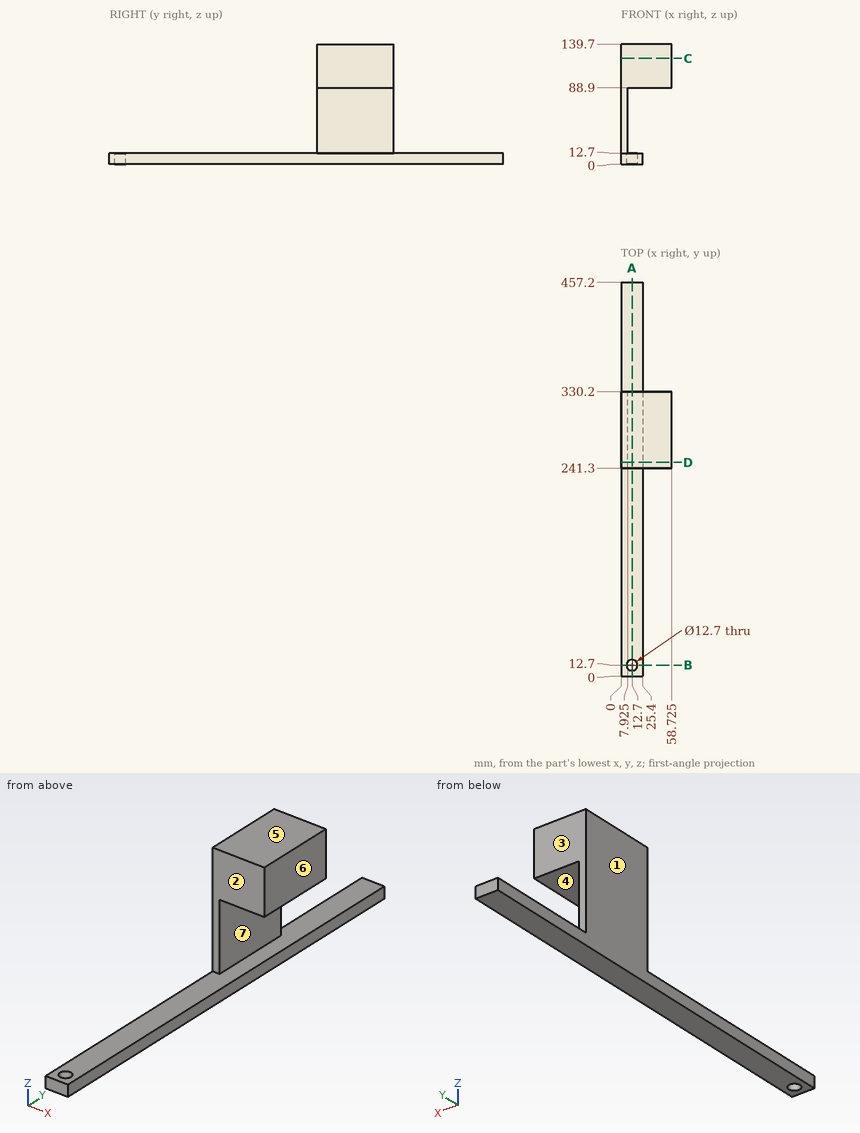
Answer from the drawing. Dimensions are ordinates in mm from the lowest x, y and z of the part. A direction names the side the tool comes from. Coordinates: 2 decimals unless noted, no trailing zeros. Write each loop counter-clockwise with the first axis right and the second up, starting at its lowest first coordinate (ties: lowest second). Pieces come first, ordered by that corner, then holes. Notation, with made-up numbers: M 46.25,7.5 L 84.25,7.5 A15 cw 84.25,27.5 Z; hole C 84.5,7.5 d5. An arc over 180 degrees is marked long. Use one line per item in the form item = value. Start each with the question number.
1. Each of these flat-tipped pins is pushed along its axis until it touches: P1, Ø4, axis at x = 27.5, z = 113.5, coming from the -Y side; P2, Ø1, axis at x = 52, z = 120.5, coming from the +Y side; P3, Ø6.5, axis at y = 216.5, z = 8.5, coming from the +X side; P4, Ø11.5, axis at x = 12.7, y = 12.7, coming from the -Z side. Where does it stop, or does it pass through?
2. The mould has two halves that part along Z. Classify the marked faces 4, 5, 6 and 7: released by +Z, released by -Z, zero draft, split by the parting line, or undercut.
3. A tool of negligible diameter and unlimited length cuts with its end or side. For the marked faces 1, 2 and 3, from which of +Z, -Z, +X, -X, +Y, -Y can it reach the whole face along a straight path? Write none if from no direction.
4. The part is cut by section A-A (x = 12.7). Give the vertices of the cut face in (y, z).
5. The part is cut by section C-C (z = 123). Give the vertices of the cut face in (x, y) (1 decimal).
6. Straight lines are drawn through the part: probe 1 along Y at (x, z) = (12, 7); probe 2 along X at (y, z) = (12, 4); probe 3 along Y at (x, z) = (21, 124.5). For each, find the intervals that lie inside material, in ascending order. Write a range as from..to.
7. The part is cut by section B-B (y = 12.7). Give the vertices of the cut face in (x, z).
8. The part is cut by section D-D (y = 248). Give the vertices of the cut face in (x, z) (1 decimal), plus the area to 3 significant figures.
Evaluation:
q1.P1 = 241.3
q1.P2 = 330.2
q1.P3 = 25.4
q1.P4 = through
q2.face_4 = undercut
q2.face_5 = released by +Z
q2.face_6 = zero draft
q2.face_7 = undercut
q3.face_1 = +Z, -Z, -X, +Y, -Y
q3.face_2 = +Z, +X, -X, -Y
q3.face_3 = +Z, +X, -X, +Y
q4.outline = M 0,0 L 6.35,0 L 6.35,12.7 L 0,12.7 Z; M 19.05,0 L 457.2,0 L 457.2,12.7 L 19.05,12.7 Z; M 241.3,88.9 L 330.2,88.9 L 330.2,139.7 L 241.3,139.7 Z
q5.outline = M 0,241.3 L 58.7,241.3 L 58.7,330.2 L 0,330.2 Z
q6.probe_1 = 0..6.39, 19.01..457.2
q6.probe_2 = 0..6.39, 19.01..25.4
q6.probe_3 = 241.3..330.2
q7.outline = M 0,0 L 6.35,0 L 6.35,12.7 L 0,12.7 Z; M 19.05,0 L 25.4,0 L 25.4,12.7 L 19.05,12.7 Z
q8.outline = M 0,0 L 25.4,0 L 25.4,12.7 L 7.9,12.7 L 7.9,88.9 L 58.7,88.9 L 58.7,139.7 L 0,139.7 Z
q8.area = 3,910 mm^2
